For this review, take the finished solid that the model builds, in its own axes (mm). Face numbers are marked on the shaded views. A direction names the side the tool comes from. Coordinates: 2 decimals unless noted, no trailing zeros. Loops run counter-clockwise (first coordinate to the right, second up) from the corner with the lowest first, then second, coordinate; pieces in that order, holes last. Notation, with made-up numbers: M 17,-13 L 35,-13 A28 ccw 35,14 Z; hole C 29,-12.5 d5. An arc over 180 degrees is marked long. Use one line per item in the form item = value.
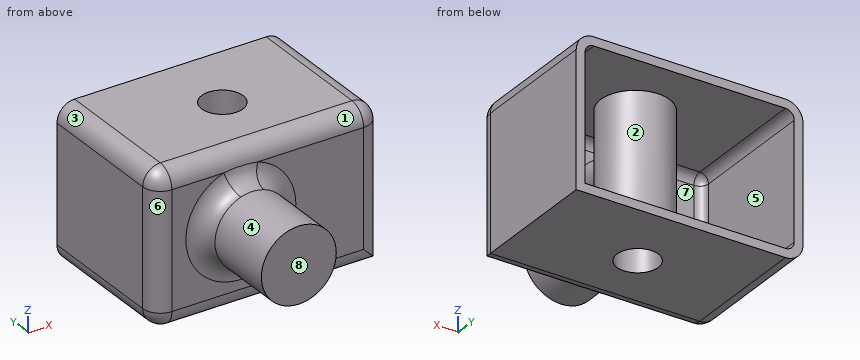
```python
from build123d import *

# Parameters (mm, degrees)
F0_W      = 65.679371357
F0_H      = 43.9539253712
F1_DEPTH  = 42.66227
F2_R      = 10.8490718956
F3_DEPTH  = 25.4
F4_R      = 5.08
F5_R      = 5.08
F6_T      = -2.54
F7_R      = 9.9976961638
F8_DEPTH  = 43.9539253712
F9_R      = 5.9952390319
F10_DEPTH = 65.60373


with BuildPart() as f1:
    # F0 (on Front) → F1 (new body)
    with BuildSketch(Plane.XZ):
        with Locations((32.8396856785, -21.9769626856)):
            Rectangle(F0_W, F0_H)
    extrude(amount=F1_DEPTH)

    # F2 (on face) → F3 (join)
    with BuildSketch(Plane.XZ.offset(42.66227)):
        with Locations((25.0557176769, -20.2263258398)):
            Circle(F2_R)
    extrude(amount=F3_DEPTH)

    # F4
    f4_edges = [f1.edges().sort_by_distance(p)[0] for p in [
        (65.679371, -42.66227, -21.976963),
        (32.839686, -42.66227, 0),
        (0, -42.66227, -21.976963),
        (32.839686, -42.66227, -43.953925),
        (65.679371, -21.331135, 0),
        (0, -21.331135, 0),
        (0, -21.331135, -43.953925),
    ]]
    fillet(f4_edges, radius=F4_R)

    # F5
    f5_edges = [f1.edges().sort_by_distance(p)[0] for p in [
        (60.599371, -42.66227, -21.976963),
        (32.839686, -42.66227, -38.873925),
        (32.839686, -42.66227, -5.08),
        (5.08, -42.66227, -21.976963),
        (14.206646, -42.66227, -20.226326),
    ]]
    fillet(f5_edges, radius=F5_R)

    # F6
    f6_openings = [f1.faces().sort_by_distance(p)[0] for p in [
        (32.90086, 0, -22.017177),
    ]]
    offset(amount=F6_T, openings=f6_openings)

    # F7 (on face) → F8 (join, through all)
    with BuildSketch(Plane(origin=(0, 0, -43.9539253712), x_dir=(1, 0, 0), z_dir=(0, 0, -1))):
        with Locations((34.7353070974, 21.0055503994)):
            Circle(F7_R)
    extrude(amount=-F8_DEPTH)

    # F9 (on face) → F10 (cut)
    with BuildSketch(Plane(origin=(0, 0, -43.9539253712), x_dir=(1, 0, 0), z_dir=(0, 0, -1))):
        with Locations((34.0243950486, 20.9764167666)):
            Circle(F9_R)
    extrude(amount=-F10_DEPTH, mode=Mode.SUBTRACT)


solid = f1.part
```
1. For pin 1 Ø5 at (x, z) = (11.5, -36.5) entering from -Y; pin 2 Ø13.5 at (x, z) = (23.5, -17) entering from +Y; pin 3 Ø4 at (x, y) = (14, -46.5) entering from +Z, all flat-tipped, find the tip position at first contact; note any pin that passes through.
Computed values:
pin_1 = -42.66
pin_2 = -12.07
pin_3 = -13.72
2. Draft analysis for pull direction X (two halves, no side actions). For the marked faces 6, 7 and 8, state which applies: +X half, -X half, draft (parallel to the pull), parting line (faces both ways), or undercut.
Computed values:
face_6 = -X half
face_7 = undercut
face_8 = draft
3. Consider section C-C on z = -37. Write out the cut boundary in (x, y).
Computed values:
outline = M 0,-37.58 A5.08 ccw 5.08,-42.66 L 60.6,-42.66 A5.08 ccw 65.68,-37.58 L 65.68,0 L 63.14,0 L 63.14,-37.58 A2.54 cw 60.6,-40.12 L 5.08,-40.12 A2.54 cw 2.54,-37.58 L 2.54,0 L 0,0 Z; C 34.74,-21.01 d20; hole C 34.02,-20.98 d11.99
4. Consider section B-B on y = -16. Write out the cut boundary in (x, z).
Computed values:
outline = M 0,-38.87 A5.08 ccw 5.08,-43.95 L 30.68,-43.95 L 30.68,0 L 5.08,0 A5.08 ccw 0,-5.08 Z; M 37.37,-43.95 L 65.68,-43.95 L 65.68,-5.08 A5.08 ccw 60.6,0 L 37.37,0 Z; hole M 2.54,-38.87 A2.54 ccw 5.08,-41.41 L 26.08,-41.41 L 26.08,-2.54 L 5.08,-2.54 A2.54 ccw 2.54,-5.08 Z; hole M 43.39,-41.41 L 63.14,-41.41 L 63.14,-5.08 A2.54 ccw 60.6,-2.54 L 43.39,-2.54 Z
5. Tool access review of the marked faces 1, 2, 3, 4 and 5: name each direction out of +Z, -Z, +X, -X, +Y, -Y from which nothing blocks a thin tool from reaching the whole face with its end or side.
Computed values:
face_1 = +Z, +X, -X, -Y
face_2 = none
face_3 = +Z, -X, +Y, -Y
face_4 = -Y
face_5 = +Y
6. Wall thickness on line 1 along Y through (x, z) = (34.5, -5.5); line 2 along X through (y, z) = (-36, -9); line 3 along Z through (x, y) = (13.5, -33): over which ranges is each line inside the solid? List them lowest first. Write a range as from..to.
Computed values:
line_1 = -42.66..-40.12, -31..-26.95, -15..-11.01
line_2 = 0..2.54, 63.14..65.68
line_3 = -43.95..-41.41, -2.54..0
7. Consider section A-A on y = -35. Write out the cut boundary in (x, z).
Computed values:
outline = M 0,-38.87 A5.08 ccw 5.08,-43.95 L 65.68,-43.95 L 65.68,-5.08 A5.08 ccw 60.6,0 L 5.08,0 A5.08 ccw 0,-5.08 Z; hole M 2.54,-38.87 A2.54 ccw 5.08,-41.41 L 63.14,-41.41 L 63.14,-5.08 A2.54 ccw 60.6,-2.54 L 5.08,-2.54 A2.54 ccw 2.54,-5.08 Z
8. Consider section D-D on x = 49. Write out the cut boundary in (y, z).
Computed values:
outline = M -42.66,-38.87 A5.08 ccw -37.58,-43.95 L 0,-43.95 L 0,-41.41 L -37.58,-41.41 A2.54 cw -40.12,-38.87 L -40.12,-5.08 A2.54 cw -37.58,-2.54 L 0,-2.54 L 0,0 L -37.58,0 A5.08 ccw -42.66,-5.08 Z
